Source: CAD feature listing. Evaluate the final solid. Frame: model axes, mm. A direction names the side the tool comes from. Coordinates: 2 decimals unless noted, no trailing zeros. Order: outer loops, then holes, each group sorted by start corner. A loop starts at its lowest first (then second) coordinate and runs counter-clockwise, first axis right, second up.
```python
from build123d import *

# Parameters (mm, degrees)
SKETCH_1_W          = 25
SKETCH_1_H          = 35
EXTRUDE_1_DEPTH     = 3
M3X0_5_1_D          = 2.5
CUT_EXTRUDE_1_DEPTH = 140.062386204


with BuildPart() as part:
    # 草图1 → 凸台-拉伸1 (new body)
    with BuildSketch(Plane.XY):
        with Locations((122.531636064, 15.602938216)):
            Rectangle(SKETCH_1_W, SKETCH_1_H)
    extrude(amount=EXTRUDE_1_DEPTH)

    # M3x0.5 螺纹孔1 (through all)
    with Locations(Plane.XY.offset(3)):
        with Locations((117.531636064, 3.5), (127.531636064, 3.5)):
            Hole(M3X0_5_1_D / 2)

    # 草图4 → 切除-拉伸1 (cut, through all)
    with BuildSketch(Plane.XY.offset(3)):
        with BuildLine():
            Line((116.631636064, 29.102938216), (116.631636064, 21.102938216))
            ThreePointArc((116.631636064, 21.102938216), (115.031636064, 19.502938216), (113.431636064, 21.102938216))
            Line((113.431636064, 21.102938216), (113.431636064, 29.102938216))
            ThreePointArc((113.431636064, 29.102938216), (115.031636064, 30.702938216), (116.631636064, 29.102938216))
        make_face()
        with BuildLine():
            Line((131.631636064, 29.102938216), (131.631636064, 21.102938216))
            ThreePointArc((131.631636064, 21.102938216), (130.031636064, 19.502938216), (128.431636064, 21.102938216))
            Line((128.431636064, 21.102938216), (128.431636064, 29.102938216))
            ThreePointArc((128.431636064, 29.102938216), (130.031636064, 30.702938216), (131.631636064, 29.102938216))
        make_face()
    extrude(amount=-CUT_EXTRUDE_1_DEPTH, mode=Mode.SUBTRACT)


solid = part.part
```
1. Section query C-C on x = 118. Return loops of the section in (y, z).
Findings:
outline: (-1.9, 0) - (2.34, 0) - (2.34, 3) - (-1.9, 3) - close; (4.66, 0) - (33.1, 0) - (33.1, 3) - (4.66, 3) - close
2. Section query A-A on y = 3.5. Return loops of the section in (x, z).
Findings:
outline: (110.03, 0) - (116.28, 0) - (116.28, 3) - (110.03, 3) - close; (118.78, 0) - (126.28, 0) - (126.28, 3) - (118.78, 3) - close; (128.78, 0) - (135.03, 0) - (135.03, 3) - (128.78, 3) - close
3. Draft query along Y for faces 1 (the face through (122, 33.103, 1)), 2 (the face through (130.067, 19.503, 1.521)), 3 (the face through (122, 16, 0)). Return one class per face: released by +Y, released by -Y, zero draft, split by the parting line, or undercut.
Findings:
face 1: released by +Y
face 2: undercut
face 3: zero draft
4. Section query B-B on z = 2.25. Return loops of the section in (x, y).
Findings:
outline: (110.03, -1.9) - (135.03, -1.9) - (135.03, 33.1) - (110.03, 33.1) - close; hole (113.43, 21.1) arc R1.6 ccw to (116.63, 21.1) - (116.63, 29.1) arc R1.6 ccw to (113.43, 29.1) - close; hole circle Ø2.5 at (117.53, 3.5); hole circle Ø2.5 at (127.53, 3.5); hole (128.43, 21.1) arc R1.6 ccw to (131.63, 21.1) - (131.63, 29.1) arc R1.6 ccw to (128.43, 29.1) - close
5. Section query D-D on y = 22.5. Return loops of the section in (x, z), plus the area to 3 significant figures.
Findings:
outline: (110.03, 0) - (113.43, 0) - (113.43, 3) - (110.03, 3) - close; (116.63, 0) - (128.43, 0) - (128.43, 3) - (116.63, 3) - close; (131.63, 0) - (135.03, 0) - (135.03, 3) - (131.63, 3) - close
area: 55.8 mm2
6. Ray query, line 1 (X direction, y = 24, z = 2.15); line 2 (X direction, y = 30, z = 0.5); line 3 (Y direction, x = 127, z = 2.15). Return the intervals inside material, ascending.
Findings:
line 1: x = 110.03 to 113.43, 116.63 to 128.43, 131.63 to 135.03
line 2: x = 110.03 to 113.71, 116.36 to 128.71, 131.36 to 135.03
line 3: y = -1.9 to 2.37, 4.63 to 33.1
7. Access query for faces 4 (the face through (122, 16, 3)), 5 (the face through (129.996, 30.703, 1.521)). Directions: +Z, -Z, +X, -X, +Y, -Y. A direction counts if a zero-diameter tool reaches every point of the face in a straight line with its end or side. Return the directions, or none.
Findings:
face 4: +Z, +X, -X, +Y, -Y
face 5: +Z, -Z
